Can you work these out from the model? Positions are in its coordinate system, mm. A direction names the side the tool comes from. Coordinates: 2 decimals unless noted, no trailing zeros. Loops run counter-clockwise (first coordinate to the right, second up) from the corner with the lowest first, then second, coordinate; pieces in that order, holes last. Notation, with made-up numbers: M 3.25,0 L 20.25,0 A6 ccw 20.25,8 Z; hole C 17.25,-31 d1. An arc over 180 degrees is marked long. Return JSON: item names as keys, results as strings. Group by question number.
```python
from build123d import *

# Parameters (mm, degrees)
F1_DEPTH = 25
F2_R     = 21
F3_DEPTH = 15
F4_R     = 20
F5_R     = 20
F6_R     = 20


with BuildPart() as f1:
    # F0 (on Top) → F1 (new body)
    with BuildSketch(Plane.XY):
        Polygon((-58.561329, 22.560807), (-108.561329, 72.560807), (-108.561329, -27.439193), align=None)
        Polygon((-8.561329, 72.560807), (-108.561329, 72.560807), (-58.561329, 22.560807), align=None)
        Polygon((-8.561329, -27.439193), (-8.561329, 72.560807), (-58.561329, 22.560807), align=None)
        Polygon((-58.561329, 22.560807), (-108.561329, -27.439193), (-8.561329, -27.439193), align=None)
    extrude(amount=F1_DEPTH)

    # F2 (on face) → F3 (cut)
    with BuildSketch(Plane.XY.offset(25)):
        with Locations((-58.561329, 22.560807)):
            Circle(F2_R)
    extrude(amount=-F3_DEPTH, mode=Mode.SUBTRACT)

    # F4
    f4_edges = [f1.edges().sort_by_distance(p)[0] for p in [
        (-108.561329, -27.439193, 12.5),
    ]]
    fillet(f4_edges, radius=F4_R)

    # F5
    f5_edges = [f1.edges().sort_by_distance(p)[0] for p in [
        (-108.561329, 72.560807, 12.5),
    ]]
    fillet(f5_edges, radius=F5_R)

    # F6
    f6_edges = [f1.edges().sort_by_distance(p)[0] for p in [
        (-8.561329, 72.560807, 12.5),
        (-8.561329, -27.439193, 12.5),
    ]]
    fillet(f6_edges, radius=F6_R)


solid = f1.part
```
1) If I drill on line 1 (Y direction, x = -58, z = 16); line 2 (Y direction, x = -65, z = 20.25); line 3 (X direction, y = 40.5, z = 20), over which ranges is the centre line in solid material (lowest first)? Write a range as from..to.
2) Suppose I cut it at B-B, the plane z = 20.75. List the corners of the cut face in (x, y) for me.
3) For pin 1 (2 mm diameter, centred on y = -11.5, z = 10.5, fed in from -X); pin 2 (4 mm diameter, centred on x = -98.5, z = 4, fed in from -Y); pin 3 (2 mm diameter, centred on y = 55.5, z = 14.5, fed in from +X); pin 4 (10 mm diameter, centred on x = -20, y = 42.5, fed in from -Z), each with a flat end and sliding along its axis, tell me the tip position at first contact or that it passes through.
4) Suppose I cut it at C-C, the plane x = -64. List the corners of the cut face in (y, z) for me.
5) For faces 4 (the face through (-59, 23, 10)), 5 (the face through (-102.858, 66.547, 12.675)), which set-ups out of +Z, -Z, +X, -X, +Y, -Y let a thin tool reach every point of the face, with its end or its side?
6) Suppose I cut it at A-A, the plane z = 5.5. List the corners of the cut face in (x, y) for me, then the cut area to 3 significant figures.
7) If we mould it in two halves opening along Y, with no side actions, what happens to faces 1 (the face through (-59, 23, 0)), 2 (the face through (-39.16, 14.52, 17.6)), 3 (the face through (-59, -27.439, 12))? For each: +Y half, -Y half, draft (parallel to the pull), parting line (faces both ways), or undercut.
8) Suppose I cut it at D-D, the plane y = -13.5. List the corners of the cut face in (x, z) for me, then the cut area to 3 significant figures.
Returned:
{
 "1": {"line 1": "y = -27.44..1.57, 43.55..72.56", "line 2": "y = -27.44..2.57, 42.55..72.56", "line 3": "x = -108.56..-69.48, -47.64..-8.56"},
 "2": {"outline": "M -108.56,-7.44 A20 ccw -88.56,-27.44 L -28.56,-27.44 A20 ccw -8.56,-7.44 L -8.56,52.56 A20 ccw -28.56,72.56 L -88.56,72.56 A20 ccw -108.56,52.56 Z; hole C -58.56,22.56 d42"},
 "3": {"pin 1": "stops at x = -108.33", "pin 2": "stops at y = -25.8", "pin 3": "stops at x = -8.66", "pin 4": "stops at z = 0"},
 "4": {"outline": "M -27.44,0 L 72.56,0 L 72.56,25 L 42.84,25 L 42.84,10 L 2.28,10 L 2.28,25 L -27.44,25 Z"},
 "5": {"face 4": "+Z", "face 5": "+Z, -Z, -X, +Y"},
 "6": {"outline": "M -108.56,-7.44 A20 ccw -88.56,-27.44 L -28.56,-27.44 A20 ccw -8.56,-7.44 L -8.56,52.56 A20 ccw -28.56,72.56 L -88.56,72.56 A20 ccw -108.56,52.56 Z", "area": "9,660 mm²"},
 "7": {"face 1": "draft", "face 2": "undercut", "face 3": "-Y half"},
 "8": {"outline": "M -107.62,0 L -9.5,0 L -9.5,25 L -107.62,25 Z", "area": "2,450 mm²"}
}
